from build123d import *

# Parameters (mm, degrees)
F0_R     = 6.1
F1_DEPTH = 25
F2_R     = 2.3
F3_DEPTH = 25
F4_DEPTH = 2
F5_D     = 3.3


with BuildPart() as f1:
    # F0 (on Top) → F1 (new body)
    with BuildSketch(Plane.XY):
        with BuildLine():
            ThreePointArc((2.75, -7.2456883731), (6.3786754111, -4.4017042154), (7.75, 0))
            ThreePointArc((7.75, 0), (-6.3786754111, 4.4017042154), (2.75, -7.2456883731))
        make_face()
        Circle(F0_R, mode=Mode.SUBTRACT)
        with BuildLine():
            Line((7.75, -16.5), (7.75, 0))
            ThreePointArc((7.75, 0), (6.3786754111, -4.4017042154), (2.75, -7.2456883731))
            Line((2.75, -7.2456883731), (2.75, -16.5))
            Line((2.75, -16.5), (7.75, -16.5))
        make_face()
    extrude(amount=F1_DEPTH)

    # F2 (on face) → F3 (cut)
    with BuildSketch(Plane(origin=(2.75, 0, 0), x_dir=(0, -1, 0), z_dir=(-1, 0, 0))):
        with BuildLine():
            ThreePointArc((7.2456883731, 17.7017590841), (8.8135894847, 18.4057690674), (9.4557512134, 20))
            ThreePointArc((9.4557512134, 20), (8.8135894847, 21.5942309326), (7.2456883731, 22.2982409159))
            Line((7.2456883731, 22.2982409159), (7.2456883731, 17.7017590841))
        make_face()
        with Locations((7.1557512134, 20)):
            Circle(F2_R)
        with Locations((7.1557512134, 10)):
            Circle(F2_R)
    extrude(amount=F3_DEPTH, mode=Mode.SUBTRACT)

    # F2 (on face) → F4 (cut)
    with BuildSketch(Plane(origin=(2.75, 0, 0), x_dir=(0, -1, 0), z_dir=(-1, 0, 0))):
        with Locations((7.1557512134, 20)):
            Circle(F2_R)
        with Locations((7.1557512134, 10)):
            Circle(F2_R)
    extrude(amount=-F4_DEPTH, mode=Mode.SUBTRACT)

    # F5 (through all)
    with Locations(Plane(origin=(2.75, 0, 0), x_dir=(0, -1, 0), z_dir=(-1, 0, 0))):
        with Locations((7.1557512134, 10), (7.1557512134, 20)):
            Hole(F5_D / 2)


solid = f1.part
Work out the finished part from the listing and answer in its coordinate system (mm). A direction names the side the tool comes from. Give positions to 0.01 mm unless a question says otherwise; leave off trailing zeros. Loops run counter-clockwise (first coordinate to the right, second up) from the corner with the lowest first, then second, coordinate; pieces in that order, holes last. Notation, with made-up numbers: M 75,75 L 122,75 A9 cw 122,83 Z; hole C 74.5,82.25 d6. An arc over 180 degrees is marked long. Use CSV: the item, a comma, the result in double quotes.
1) Find section D-D on y = -6.5. Write down the section's boundary in (x, z), plus the area to 3 significant figures.
Answer:
outline,"M -4.22,0 L 7.75,0 L 7.75,8.49 L 4.75,8.49 L 4.75,7.8 L -4.22,7.8 Z; M -4.22,12.2 L 4.75,12.2 L 4.75,11.51 L 7.75,11.51 L 7.75,18.49 L 4.75,18.49 L 4.75,17.8 L -4.22,17.8 Z; M -4.22,22.2 L 4.75,22.2 L 4.75,21.51 L 7.75,21.51 L 7.75,25 L -4.22,25 Z"
area,"202 mm^2"
2) Consider L1, parallel to Z at x = 6, y = -7; L2, parallel to X at y = -10.5, z = 13.25; L3, parallel to X at y = -1.75, z = 8. Determine where each line is inside the solid, lowest interval first.
Answer:
L1,"0 to 8.36, 11.64 to 18.36, 21.64 to 25"
L2,"2.75 to 7.75"
L3,"-7.55 to -5.84, 5.84 to 7.75"
3) Which of the six approach directions +Z, -Z, +X, -X, +Y, -Y give full straight-line access (tool end or side, diameter ignored) to faces 4 (the flat face through (2, -6, 25)), 5 (the flat face through (4.75, -7, 22))?
Answer:
face 4,"+Z, +X, -X, +Y, -Y"
face 5,"-X"
4) Determine the mould class of faces 1 (the flat face through (5, -16.5, 12)), 2 (the flat face through (4.75, -7, 12)), 3 (the flat face through (2, -6, 0)) for opening direction Y: released by +Y, released by -Y, zero draft, split by the parting line, or undercut.
Answer:
face 1,"released by -Y"
face 2,"undercut"
face 3,"zero draft"
5) Given P1, Ø7.5, axis at x = 0, y = 0, coming from the +Z side; P2, Ø1.5, axis at x = 0, z = 13.5, coming from the -Y side; P3, Ø5, axis at x = -5.5, z = 19, coming from the +Y side; P4, Ø4, axis at y = -7.16, z = 20, coming from the -X side, each flat-ended and moving along its own axis, determine where each tip first touches the part or whether it passes through.
Answer:
P1,"through"
P2,"y = -7.75"
P3,"y = 7.15"
P4,"x = 4.75"
6) Find section B-B on z = 15.25. Write down the section's boundary in (x, y), plus the area to 3 significant figures.
Answer:
outline,"M 2.75,-16.5 L 7.75,-16.5 L 7.75,0 A7.75 ccw long 2.75,-7.25 Z; hole C 0,0 d12.2"
area,"128 mm^2"
7) Find section A-A on y = -0.5. Write down the section's boundary in (x, z).
Answer:
outline,"M -7.73,0 L -6.08,0 L -6.08,25 L -7.73,25 Z; M 6.08,0 L 7.75,0 L 7.75,25 L 6.08,25 Z"
8) Find section C-C on x = -2. Write down the section's boundary in (y, z), plus the area to 3 significant figures.
Answer:
outline,"M -7.49,0 L -5.76,0 L -5.76,8.17 A2.3 cw -7.49,7.72 Z; M -7.49,12.28 A2.3 cw -5.76,11.83 L -5.76,18.17 A2.3 cw -7.49,17.72 Z; M -7.49,22.28 A2.3 cw -5.76,21.83 L -5.76,25 L -7.49,25 Z; M 5.76,0 L 7.49,0 L 7.49,25 L 5.76,25 Z"
area,"71.2 mm^2"
